```python
from build123d import *

# Parameters (mm, degrees)
F1_DEPTH    = 10
F2_W        = 180
F2_H        = 70
F3_DEPTH    = 10.001
F4_T1_DEPTH = 120.3455223822
F5_R        = 5
F6_T1_DEPTH = 541.5885597996
F7_R        = 10
F9_D        = 3.2
F9_DEPTH    = 6
F9_TIP      = 0.9613769904
F11_D       = 10


# Not quite as in the source:
# - a fillet or chamfer that OpenCascade refuses, or shapes differently, is made with other operations: its cross-section is extruded or revolved along the edge and cut away or added


with BuildPart() as f1:
    # F0 (on Front) → F1 (new body)
    with BuildSketch(Plane.XZ):
        with BuildLine():
            Line((-30, 578), (0, 0))
            Line((0, 0), (500, 0))
            Line((500, 0), (530, 578))
            ThreePointArc((530, 578), (250, 605), (-30, 578))
        make_face()
    extrude(amount=F1_DEPTH)

    # F2 (on face) → F3 (cut, through all)
    with BuildSketch(Plane.XZ.offset(10)):
        with Locations((250, 475)):
            Rectangle(F2_W, F2_H)
    extrude(amount=-F3_DEPTH, mode=Mode.SUBTRACT)

    # F4: fillet of radius 25 on 2 edges, made by hand

    # F4_s2 → F4_t1 (cut)
    with BuildSketch(Plane.XZ.offset(-55.1727611911)):
        with BuildLine():
            add(Edge.make_bspline(
                [(-28.865884536, 556.1493753933), (-30.0086821523, 578.1672761351), (-8.3063912994, 582.0537283993)],
                knots=[0, 0, 0, 1, 1, 1], degree=2, weights=[1, 1, 1]))
            ThreePointArc((-8.3063912994, 582.0537283993), (-19.1608272147, 580.0677046728), (-30, 578))
            Line((-30, 578), (-28.865884536, 556.1493753933))
        make_face()
        with BuildLine():
            add(Edge.make_bspline(
                [(508.3063912994, 582.0537283993), (530.0086821523, 578.1672761351), (528.865884536, 556.1493753933)],
                knots=[0, 0, 0, 1, 1, 1], degree=2, weights=[1, 1, 1]))
            Line((528.865884536, 556.1493753933), (530, 578))
            ThreePointArc((530, 578), (519.1608272147, 580.0677046728), (508.3063912994, 582.0537283993))
        make_face()
    extrude(amount=F4_T1_DEPTH, mode=Mode.SUBTRACT)

    # F5
    f5_edges = [f1.edges().sort_by_distance(p)[0] for p in [
        (500, -5, 0),
        (0, -5, 0),
    ]]
    fillet(f5_edges, radius=F5_R)

    # F6: chamfer of 5.7 x 9.8726896031 on 1 edges, made by hand

    # F6_s2 → F6_t1 (cut)
    with BuildSketch(Plane.YZ.offset(-20.7942798998)):
        Polygon((-10, 5.7), (-0.1273103969, 0), (-10, 0), align=None)
    extrude(amount=F6_T1_DEPTH, mode=Mode.SUBTRACT)

    # F7
    f7_edges = [f1.edges().sort_by_distance(p)[0] for p in [
        (340, -5, 510),
        (160, -5, 510),
        (160, -5, 440),
        (340, -5, 440),
    ]]
    fillet(f7_edges, radius=F7_R)

    # F9
    with Locations(Plane.XZ.offset(10)):
        with Locations((150, 525), (200, 525), (250, 525), (250, 425), (200, 425), (150, 425), (150, 475), (350, 525), (350, 475), (350, 425), (300, 425), (300, 525)):
            Hole(F9_D / 2, depth=F9_DEPTH)
            with Locations((0, 0, -(F9_DEPTH + F9_TIP / 2))):  # 118° drill point
                Cone(0, F9_D / 2, F9_TIP, mode=Mode.SUBTRACT)

    # F11 (through all)
    with Locations(Plane.XZ.offset(10)):
        with Locations((480, 555), (502, 555)):
            Hole(F11_D / 2)


solid = f1.part
```
Design review of the part built by this model. Coordinates are the model's own, in mm. Give positions to 0.01 mm unless a question says otherwise; leave off trailing zeros. Order: outer loops, then holes, each group sorted by start corner. A loop starts at its lowest first (then second) coordinate and runs counter-clockwise, first axis right, second up. Notation, with made-up numbers: (-4, 55.25) -> (36, 55.25) arc R13 cw to (36, 76.25) -> close; hole circle Ø8 at (58.5, -22.5). An arc over 180 degrees is marked (long way). Write item = value, one per line. Start each with the question number.
(1) We need section A-A on x = 287. Write out the cut boundary in (y, z).
(2) For pin 1 (1 mm diameter, centred on y = -7.5, z = 454.5, fed in from -X); pin 2 (1 mm diameter, centred on y = -7.5, z = 457, fed in from -X); pin 3 (1.9 mm diameter, centred on x = 300, z = 425, fed in from -Y), all flat-tipped, find the tip position at first contact; note any pin that passes through.
(3) We need section B-B on x = 93. Write out the cut boundary in (y, z).
(4) We need section D-D on x = 187. Write out the cut boundary in (y, z), plus the area to 3 significant figures.
(5) To check wall thickness, follow line 1 along Z through (x, y) = (250.5, -5); line 2 along X through (y, z) = (-7.2, 425); line 3 along Z through (x, y) = (250, -8.7). State the ranges of each line that lie inside material, in increasing order.
(6) We need section C-C on y = -6.5. State how many separate pieces and enclosed holes the cut face has, plus the area to 3 significant figures.
Numbers:
q1.outline = (-10, 5.7) -> (-0.13, 0) -> (0, 0) -> (0, 440) -> (-10, 440) -> close; (-10, 510) -> (0, 510) -> (0, 604.53) -> (-10, 604.53) -> close
q2.pin_1 = -23.62
q2.pin_2 = -23.75
q2.pin_3 = -3.61
q3.outline = (-10, 5.7) -> (-0.13, 0) -> (0, 0) -> (0, 596.57) -> (-10, 596.57) -> close
q4.outline = (-10, 5.7) -> (-0.13, 0) -> (0, 0) -> (0, 440) -> (-10, 440) -> close; (-10, 510) -> (0, 510) -> (0, 603.65) -> (-10, 603.65) -> close
q4.area = 5,310 mm^2
q5.line_1 = 2.81 to 423.48, 426.52 to 440, 510 to 523.48, 526.52 to 605
q5.line_2 = -22.06 to 148.4, 151.6 to 198.4, 201.6 to 248.4, 251.6 to 298.4, 301.6 to 348.4, 351.6 to 522.06
q5.line_3 = 4.95 to 423.4, 426.6 to 440, 510 to 523.4, 526.6 to 605
q6.separate_pieces = 1
q6.enclosed_holes = 15
q6.area = 302,000 mm^2
